The model under review builds one solid part; all positions refer to its coordinate system, in mm. Face numbers are marked on the shaded views. Coordinates: 2 decimals unless noted, no trailing zeros. Loops run counter-clockwise (first coordinate to the right, second up) from the corner with the lowest first, then second, coordinate; pieces in that order, holes last. Notation, with made-up numbers: M 77,82 L 132,82 A18 cw 132,111 Z; hole C 64,28.5 d1. An arc over 180 degrees is marked long. Use one line per item in the form item = value.
```python
from build123d import *

# Parameters (mm, degrees)
SKETCH_1_W          = 47
SKETCH_1_H          = 23
EXTRUDE_1_DEPTH     = 3
SKETCH_2_R          = 1.6
SKETCH_2_R_2        = 6.75
CUT_EXTRUDE_1_DEPTH = 27.334388165
FILLET_1_R          = 10


with BuildPart() as part:
    # 草图1 → 凸台-拉伸1 (new body)
    with BuildSketch(Plane(origin=(0, 0, 0), x_dir=(1, 0, 0), z_dir=(0, 1, 0))):
        Rectangle(SKETCH_1_W, SKETCH_1_H)
    extrude(amount=EXTRUDE_1_DEPTH)

    # 草图2 → 切除-拉伸1 (cut, through all)
    with BuildSketch(Plane(origin=(0, 3, 0), x_dir=(1, 0, 0), z_dir=(0, 1, 0))):
        with Locations(Location((-19.727241336, 6.25, 0), (0, 0, 270))):
            Circle(SKETCH_2_R)
        with Locations(Location((-11.5, -8, 0), (0, 0, 270))):
            Circle(SKETCH_2_R)
        with Locations(Location((-3.272758664, 6.25, 0), (0, 0, 270))):
            Circle(SKETCH_2_R)
        with Locations(Location((-11.5, 1.5, 0), (0, 0, 270))):
            Circle(SKETCH_2_R_2)
        with Locations(Location((18.5, 7.75, 0), (0, 0, 270))):
            Circle(SKETCH_2_R)
        with Locations(Location((18.5, 0.25, 0), (0, 0, 270))):
            Circle(SKETCH_2_R)
        with Locations(Location((8.5, 0.25, 0), (0, 0, 90))):
            Circle(SKETCH_2_R)
        with Locations(Location((8.5, 7.75, 0), (0, 0, 90))):
            Circle(SKETCH_2_R)
    extrude(amount=-CUT_EXTRUDE_1_DEPTH, mode=Mode.SUBTRACT)

    # 圆角1
    fillet_1_edges = [part.edges().sort_by_distance(p)[0] for p in [
        (23.5, 1.5, 11.5),
    ]]
    fillet(fillet_1_edges, radius=FILLET_1_R)


solid = part.part
```
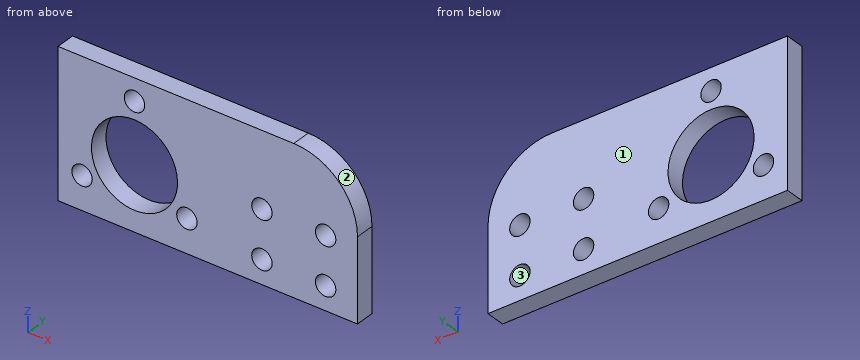
1. Add section D-D (y = 2.5). Count the separate pieces of the cut face and the enclosed holes in it, then the cut area to 3 significant figures.
Response values:
separate_pieces = 1
enclosed_holes = 8
area = 860 mm^2
2. Wall thickness on line 1 along Z through (x, y) = (8.5, 1.1); line 2 along X through (y, z) = (2.2, -0.25); line 3 along X through (y, z) = (2.55, -0.5): over which ranges is each line inside the solid? List them lowest first. Write a range as from..to.
Response values:
line_1 = -11.5..-9.35, -6.15..-1.85, 1.35..11.5
line_2 = -23.5..-18.13, -4.87..6.9, 10.1..16.9, 20.1..23.5
line_3 = -23.5..-18.18, -4.82..6.92, 10.08..16.92, 20.08..23.5
3. Add section C-C (x = 18.5). State the section outline as (y, z) points, then the cut area to 3 significant figures.
Response values:
outline = M 0,-11.5 L 3,-11.5 L 3,-9.35 L 0,-9.35 Z; M 0,-6.15 L 3,-6.15 L 3,-1.85 L 0,-1.85 Z; M 0,1.35 L 3,1.35 L 3,10.16 L 0,10.16 Z
area = 45.8 mm^2
4. Add section B-B (z = 8.75). State the section outline as (x, y) points, then the cut area to 3 significant figures.
Response values:
outline = M -23.5,0 L -12.91,0 L -12.91,3 L -23.5,3 Z; M -10.09,0 L 20.39,0 L 20.39,3 L -10.09,3 Z
area = 123 mm^2
5. The part is to be moulded in two halves that separate along X. For the marked faces 1, 2 and 3, say which applies: pulls with the +X half, pulls with the -X half, needs draft (parallel to the pull), parting line crosses it, or undercut.
Response values:
face_1 = needs draft
face_2 = pulls with the +X half
face_3 = undercut
6. Add section A-A (x = -16.5). State the section outline as (y, z) points, then the cut area to 3 significant figures.
Response values:
outline = M 0,-11.5 L 3,-11.5 L 3,-6.03 L 0,-6.03 Z; M 0,3.03 L 3,3.03 L 3,11.5 L 0,11.5 Z
area = 41.8 mm^2
